Verification items for the finished model (mm, model axes). A direction names the side the tool comes from. Coordinates: 2 decimals unless noted, no trailing zeros. Loops run counter-clockwise (first coordinate to the right, second up) from the corner with the lowest first, then second, coordinate; pieces in that order, holes last. Notation, with made-up numbers: (-17.75, 34) -> (-13.75, 34) arc R34 ccw to (-13.75, 72) -> close; hole circle Ø2 at (72.25, 38). An arc over 180 degrees is marked (long way). Use CSV: the item, a comma, the result in double quotes. Start each with the question number.
Autodesk Inventor part; units mm, degrees
ref_plane "YZ Plane" through (0, 0, 0) normal (1, 0, 0) x (0, 1, 0)
ref_plane "XZ Plane" through (0, 0, 0) normal (0, 1, 0) x (-1, 0, 0)
ref_plane "XY Plane" through (0, 0, 0) normal (0, 0, 1) x (1, 0, 0)
sketch "Sketch2" plane through (0, 0, 0) normal (0, 1, 0) x (-1, 0, 0)
  line L0 (-18.5, 18.5) -> (18.5, 18.5)
  line L1 (18.5, 18.5) -> (18.5, -18.5)
  line L2 (18.5, -18.5) -> (-18.5, -18.5)
  line L3 (-18.5, -18.5) -> (-18.5, 18.5)
  line L4 (-18.5, 18.5) -> (18.5, -18.5) construction
  line L5 (18.5, 18.5) -> (-18.5, -18.5) construction
  line L6 (12, -14.5) -> (18, -14.5)
  line L7 (18, -14.5) -> (18, -5.5)
  line L8 (18, -5.5) -> (12, -5.5)
  line L9 (12, -5.5) -> (12, -14.5)
  line L10 (12, -14.5) -> (18, -5.5) construction
  line L11 (18, -14.5) -> (12, -5.5) construction
  line L12 (0, 18.5) -> (0, -18.5) construction
  line L13 (18.5, 0) -> (-18.5, 0) construction
  circle A0 centre (0, 0) radius 3
  circle A1 centre (6, -6) radius 2.5
  circle A2 centre (-6, 6) radius 2.5
  circle A3 centre (3, -7.953) radius 1
  line L14 (12, 14.5) -> (18, 14.5)
  line L15 (18, 14.5) -> (18, 5.5)
  line L16 (18, 5.5) -> (12, 5.5)
  line L17 (12, 5.5) -> (12, 14.5)
  line L18 (12, 14.5) -> (18, 5.5) construction
  line L19 (18, 14.5) -> (12, 5.5) construction
  line L20 (-12, -14.5) -> (-18, -14.5)
  line L21 (-18, -14.5) -> (-18, -5.5)
  line L22 (-18, -5.5) -> (-12, -5.5)
  line L23 (-12, -5.5) -> (-12, -14.5)
  line L24 (-12, -14.5) -> (-18, -5.5) construction
  line L25 (-18, -14.5) -> (-12, -5.5) construction
  line L26 (-12, 5.5) -> (-12, 14.5)
  line L27 (-12, 14.5) -> (-18, 14.5)
  line L28 (-18, 14.5) -> (-18, 5.5)
  line L29 (-12, 14.5) -> (-18, 5.5) construction
  line L30 (-18, 14.5) -> (-12, 5.5) construction
  line L31 (-18, 5.5) -> (-12, 5.5)
  circle A4 centre (6, 6) radius 2.5
  circle A5 centre (-6, -6) radius 2.5
  circle A6 centre (3, 7.953) radius 1
  point P0 (15, -10)
  point P1 (15, 10)
  point P2 (-15, -10)
  point P3 (-15, 10)
  dimension "d0" = 37
  dimension "d1" = 37
  dimension "d3" = 9
  dimension "d5" = 6
  dimension "d8" = 5
  dimension "d10" = 6
  dimension "d11" = 6
  dimension "d23" = 2
  dimension "d27" = 6
  dimension "d30" = 15
  dimension "d32" = 14.5
  dimension "d33" = 9
  dimension "d35" = 8.5
extrude "Extrusion1" add sketch "Sketch2" along normal blind 6
equation "\"d0\" = d1"
equation "\"d11\" = d10"
properties part number "thumper-base-v3"
1. Scan lines: line 1 (Z direction, x = 16.5, y = 2.1); line 2 (X direction, y = 3.25, z = 12); line 3 (Z direction, x = -6, y = 2.05). Record each from-to range of solid material in increasing order.
2. Depth check by flat-ended pin: pin 1 (6 mm diameter, centred on x = 0, z = 8, fed in from -Y); pin 2 (1.2 mm diameter, centred on x = -3, z = 7.953, fed in from -Y). Enter the tip coordinate at first touch or a pass-through.
3. Release check for a two-part mould opening along Z. For faces 3 (the flat face through (18, 3, -10)), 4 (the flat face through (0, 3, -18.5)), 5 (the flat face through (0, 6, 4)), 6 (the cylindrical face through (-2.87, 2.958, -8.944)) record: released by +Z, released by -Z, zero draft, split by the parting line, or undercut.
4. Cross-section at C-C, the plane z = -6. Record the boundary of the cut face in (x, y).
5. Cross-section at D-D, the plane x = -6. Record the boundary of the cut face in (y, z).
6. Cross-section at B-B, the plane x = 0. Record the boundary of the cut face in (y, z), plus the area to 3 significant figures.
7. Set-up check for faces 1 (the flat face through (0, 0, 4)), 2 (the flat face through (-12, 3, -10)): record each of +Z, -Z, +X, -X, +Y, -Y from which the full face is reachable in a straight line by a thin tool's end or side.
8. Cross-section at A-A, the plane z = -12. Record the boundary of the cut face in (x, y), plus the area to 3 significant figures.
Solution:
1,line 1,"z = -18.5 to -14.5, -5.5 to 5.5, 14.5 to 18.5"
1,line 2,"x = -18.5 to -18, -12 to 12, 18 to 18.5"
1,line 3,"z = -18.5 to -8.5, -3.5 to 3.5, 8.5 to 18.5"
2,pin 1,"stops at y = 0"
2,pin 2,"passes through"
3,face 3,"undercut"
3,face 4,"released by -Z"
3,face 5,"zero draft"
3,face 6,"undercut"
4,outline,"(-18.5, 0) -> (-18, 0) -> (-18, 6) -> (-18.5, 6) -> close; (-12, 0) -> (-8.5, 0) -> (-8.5, 6) -> (-12, 6) -> close; (-3.5, 0) -> (3.5, 0) -> (3.5, 6) -> (-3.5, 6) -> close; (8.5, 0) -> (12, 0) -> (12, 6) -> (8.5, 6) -> close; (18, 0) -> (18.5, 0) -> (18.5, 6) -> (18, 6) -> close"
5,outline,"(0, -18.5) -> (6, -18.5) -> (6, -8.5) -> (0, -8.5) -> close; (0, -3.5) -> (6, -3.5) -> (6, 3.5) -> (0, 3.5) -> close; (0, 8.5) -> (6, 8.5) -> (6, 18.5) -> (0, 18.5) -> close"
6,outline,"(0, -18.5) -> (6, -18.5) -> (6, -3) -> (0, -3) -> close; (0, 3) -> (6, 3) -> (6, 18.5) -> (0, 18.5) -> close"
6,area,"186 mm2"
7,face 1,"+Z, -Z, +X, -X, -Y"
7,face 2,"+Y, -Y"
8,outline,"(-18.5, 0) -> (-18, 0) -> (-18, 6) -> (-18.5, 6) -> close; (-12, 0) -> (12, 0) -> (12, 6) -> (-12, 6) -> close; (18, 0) -> (18.5, 0) -> (18.5, 6) -> (18, 6) -> close"
8,area,"150 mm2"
